Check sheet for the modelled part. Datum: model origin and axes. Units: mm. A direction names the side the tool comes from. Give positions to 0.01 mm unless a question says otherwise; leave off trailing zeros. Write each loop counter-clockwise with the first axis right and the second up, starting at its lowest first coordinate (ties: lowest second). Pieces come first, ordered by that corner, then holes. Notation, with made-up numbers: (76.5, 70) -> (132.5, 70) arc R20 ccw to (132.5, 109) -> close; hole circle Ø11 at (24, 77). An arc over 180 degrees is marked (long way). Use a Markdown table: item, result. Add a question column.
1. Cross-section at C-C (y = 7.5). Enter the section's corners in (x, z), then the cut area to 3 significant figures.
2. Cross-section at A-A (x = 3.75). Enter the section's corners in (y, z).
3. Cross-section at D-D (x = -4.75). Enter the section's corners in (y, z).
4. Release check for a two-part mould opening along Y. For faces 3 (the cylindrical face through (5.9, 0.39, 0.09)), 4 (the cylindrical face through (-4.759, 6.025, 0.089)), 5 (the flat face through (0, 1.27, 0)), 6 (the flat face through (0, 1, 6.35)) record: released by +Y, released by -Y, zero draft, split by the parting line, or undercut.
5. Set-up check for faces 1 (the flat face through (-4.77, 3.39, 0.09)), 2 (the flat face through (0, 1, -6.35)): record each of +Z, -Z, +X, -X, +Y, -Y from which the full face is reachable in a straight line by a thin tool's end or side.
6. Scan lines: probe 1 along Y at (x, z) = (-2, -3.75); probe 2 along Y at (x, z) = (-3.25, 4.5); probe 3 along X at (y, z) = (2.25, -5.25). Record each from-to range of solid material in increasing order. Write a range as [from, to].
7. Gauge pin test, flat ends, axial feed: P1, Ø1, axis at y = 2.5, z = -2.5, coming from the -X side; P2, Ø1.5, axis at y = 2.5, z = 4.5, coming from the +X side; P3, Ø2, axis at x = -5, z = -0.5, coming from the +Y side; P4, Ø0.6, axis at x = 1, y = -0.5, coming from the +Z side. Record the tip position at first contact, or that the pin passes through.
from build123d import *

# Parameters (mm, degrees)
BOSS_EXTRUDE3_DEPTH      = 6.35
BOSS_EXTRUDE3_DEPTH_BACK = 6.35
SKETCH6_W                = 9.8425
SKETCH6_H                = 11.938
BOSS_EXTRUDE4_DEPTH      = 0.762


with BuildPart() as part:
    # Sketch5 → Boss-Extrude3 (new body, two sides)
    with BuildSketch(Plane.XY) as boss_extrude3_sk:
        with BuildLine():
            Line((-4.92125, 0), (4.92125, 0))
            ThreePointArc((4.92125, 0), (5.908287619, 0.395752758), (6.348521584, 1.363770094))
            ThreePointArc((6.348521584, 1.363770094), (3.976448154, 7.693025011), (-2.238375, 10.3505))
            ThreePointArc((-2.238375, 10.3505), (-4.696720113, 9.332220113), (-5.715, 6.873875))
            ThreePointArc((-5.715, 6.873875), (-5.08, 6.238875), (-4.445, 6.873875))
            ThreePointArc((-4.445, 6.873875), (-3.798694501, 8.434194501), (-2.238375, 9.0805))
            ThreePointArc((-2.238375, 9.0805), (3.058228384, 6.815658238), (5.079835732, 1.42153001))
            ThreePointArc((5.079835732, 1.42153001), (5.030920847, 1.313972529), (4.92125, 1.27))
            Line((4.92125, 1.27), (-4.92125, 1.27))
            ThreePointArc((-4.92125, 1.27), (-5.042012288, 1.325706163), (-5.078022403, 1.453729514))
            Line((-5.078022403, 1.453729514), (-4.452910387, 5.376956946))
            ThreePointArc((-4.452910387, 5.376956946), (-4.980081946, 6.103964613), (-5.707089613, 5.576793054))
            Line((-5.707089613, 5.576793054), (-6.332201629, 1.653565622))
            ThreePointArc((-6.332201629, 1.653565622), (-6.00811059, 0.501355466), (-4.92125, 0))
        make_face()
    extrude(amount=BOSS_EXTRUDE3_DEPTH)
    extrude(boss_extrude3_sk.sketch, amount=-BOSS_EXTRUDE3_DEPTH_BACK)

    # Sketch6 → Boss-Extrude4 (add)
    with BuildSketch(Plane.XZ):
        Rectangle(SKETCH6_W, SKETCH6_H)
    extrude(amount=BOSS_EXTRUDE4_DEPTH)


solid = part.part
Worked answers:
| question | item | result |
|---|---|---|
| 1 | outline | (-5.66, -6.35) -> (-4.35, -6.35) -> (-4.35, 6.35) -> (-5.66, 6.35) -> close; (2.31, -6.35) -> (4.16, -6.35) -> (4.16, 6.35) -> (2.31, 6.35) -> close |
| 1 | area | 40.0 mm² |
| 2 | outline | (-0.76, -5.97) -> (0, -5.97) -> (0, -6.35) -> (1.27, -6.35) -> (1.27, 6.35) -> (0, 6.35) -> (0, 5.97) -> (-0.76, 5.97) -> close; (5.97, -6.35) -> (7.92, -6.35) -> (7.92, 6.35) -> (5.97, 6.35) -> close |
| 3 | outline | (-0.76, -5.97) -> (0, -5.97) -> (0, -6.35) -> (1.27, -6.35) -> (1.27, 6.35) -> (0, 6.35) -> (0, 5.97) -> (-0.76, 5.97) -> close; (3.51, -6.35) -> (6.02, -6.35) -> (6.02, 6.35) -> (3.51, 6.35) -> close; (6.33, -6.35) -> (9.28, -6.35) -> (9.28, 6.35) -> (6.33, 6.35) -> close |
| 4 | face 3 | released by -Y |
| 4 | face 4 | undercut |
| 4 | face 5 | undercut |
| 4 | face 6 | zero draft |
| 5 | face 1 | +Z, -Z |
| 5 | face 2 | -Z, +X, -X, +Y, -Y |
| 6 | probe 1 | y = [-0.76, 1.27], [9.08, 10.35] |
| 6 | probe 2 | y = [-0.76, 1.27], [8.83, 10.2] |
| 6 | probe 3 | x = [-6.24, -4.95], [5.07, 6.34] |
| 7 | P1 | stops at x = -6.28 |
| 7 | P2 | stops at x = 6.36 |
| 7 | P3 | stops at y = 9.87 |
| 7 | P4 | stops at z = 5.97 |
